from build123d import *

# Parameters (mm, degrees)
SKETCH1_R      = 2.38252
EXTRUDE1_DEPTH = 3.175
EXTRUDE2_DEPTH = 3.175
CHAMFER1_SIZE  = 6.35


with BuildPart() as part:
    # Sketch1 → Extrude1 (new body)
    with BuildSketch(Plane(origin=(0, 0, 0), x_dir=(1, 0, 0), z_dir=(0, 1, 0))):
        with BuildLine():
            Line((-31.75, 28.575), (31.75, 28.575))
            ThreePointArc((31.75, 28.575), (38.485192091, 25.785192091), (41.275, 19.05))
            Line((41.275, 19.05), (41.275, -19.05))
            ThreePointArc((41.275, -19.05), (38.485192091, -25.785192091), (31.75, -28.575))
            Line((31.75, -28.575), (-31.75, -28.575))
            ThreePointArc((-31.75, -28.575), (-38.485192091, -25.785192091), (-41.275, -19.05))
            Line((-41.275, -19.05), (-41.275, 19.05))
            ThreePointArc((-41.275, 19.05), (-38.485192091, 25.785192091), (-31.75, 28.575))
        make_face()
        with Locations(Location((38.1, 0, 0), (0, 0, 270))):
            Circle(SKETCH1_R, mode=Mode.SUBTRACT)
        with Locations(Location((-38.1, 0, 0), (0, 0, 90))):
            Circle(SKETCH1_R, mode=Mode.SUBTRACT)
    extrude(amount=EXTRUDE1_DEPTH)

    # Sketch2 → Extrude2 (add)
    with BuildSketch(Plane(origin=(0, 0, 0), x_dir=(1, 0, 0), z_dir=(0, 1, 0))):
        Polygon((31.75, 28.575), (41.275, 19.05), (41.275, 28.575), align=None)
        Polygon((-31.75, 28.575), (-41.275, 19.05), (-41.275, 28.575), align=None)
        Polygon((-41.275, -19.05), (-31.75, -28.575), (-41.275, -28.575), align=None)
        Polygon((41.275, -19.05), (31.75, -28.575), (41.275, -28.575), align=None)
    extrude(amount=EXTRUDE2_DEPTH)

    # Chamfer1
    chamfer1_edges = [part.edges().sort_by_distance(p)[0] for p in [
        (41.275, 1.5875, -28.575),
        (-41.275, 1.5875, -28.575),
        (-41.275, 1.5875, 28.575),
        (41.275, 1.5875, 28.575),
    ]]
    chamfer(chamfer1_edges, length=CHAMFER1_SIZE)


solid = part.part
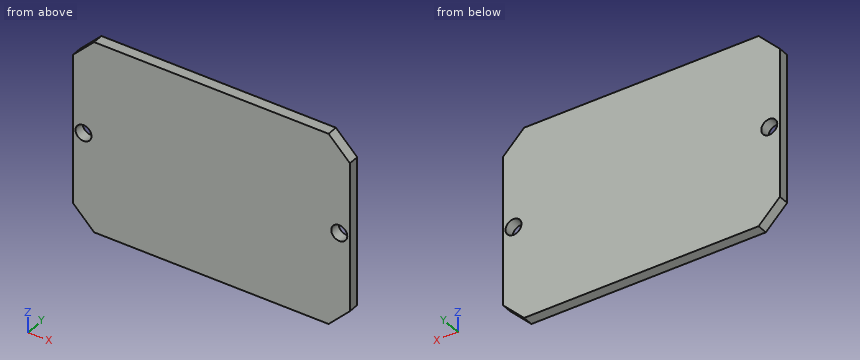
Model file for the job. Use its own axes, mm. Give positions to 0.01 mm unless a question says otherwise; leave off trailing zeros. Loops run counter-clockwise (first coordinate to the right, second up) from the corner with the lowest first, then second, coordinate; pieces in that order, holes last.
1) Wall check: line 1 (X direction, y = 1.25, z = 0) (3 decimals); line 2 (X direction, y = 0.25, z = -2) (3 decimals); line 3 (Z direction, x = -38.1, y = 1.2). Give the ranges that are in metal, low to high.
2) Saw through at C-C (x = 38.1). Write the cut outline in (y, z) (3 decimals), plus the area to 3 significant figures.
3) Saw through at B-B (y = 0.9). Write the cut outline in (x, z) (3 decimals).
4) Saw through at A-A (z = 0). Write the cut outline in (x, y) (3 decimals).
Answer block:
1. line 1: x = -41.275 to -40.483, -35.717 to 35.717, 40.483 to 41.275
1. line 2: x = -41.275 to -39.395, -36.805 to 36.805, 39.395 to 41.275
1. line 3: z = -25.4 to -2.38, 2.38 to 25.4
2. outline: (0, -25.4) - (3.175, -25.4) - (3.175, -2.383) - (0, -2.383) - close; (0, 2.383) - (3.175, 2.383) - (3.175, 25.4) - (0, 25.4) - close
2. area: 146 mm2
3. outline: (-41.275, -22.225) - (-34.925, -28.575) - (34.925, -28.575) - (41.275, -22.225) - (41.275, 22.225) - (34.925, 28.575) - (-34.925, 28.575) - (-41.275, 22.225) - close; hole circle Ø4.765 at (-38.1, 0); hole circle Ø4.765 at (38.1, 0)
4. outline: (-41.275, 0) - (-40.483, 0) - (-40.483, 3.175) - (-41.275, 3.175) - close; (-35.717, 0) - (35.717, 0) - (35.717, 3.175) - (-35.717, 3.175) - close; (40.483, 0) - (41.275, 0) - (41.275, 3.175) - (40.483, 3.175) - close
